Read the model definition and answer for the solid it produces. Units are mm, in the model's axes. A direction names the side the tool comes from. Give positions to 0.01 mm unless a question says otherwise; leave off trailing zeros. Write each loop counter-clockwise with the first axis right and the second up, starting at its lowest first coordinate (ties: lowest second). Pieces come first, ordered by that corner, then holes. Notation, with made-up numbers: (58, 66) - (66, 66) arc R32 ccw to (66, 100) - close; hole circle Ø11 at (-4.75, 76). An arc over 180 degrees is marked (long way). Answer as CSV lines item,"result".
```python
from build123d import *

# Parameters (mm, degrees)
F1_DEPTH      = 15
F2_W          = 70
F2_H          = 12
F3_DEPTH      = 10
F4_R          = 1.375
F4_R_2        = 1
F5_DEPTH      = 25
F5_DEPTH_BACK = 25
F6_R          = 1
F7_DEPTH      = 10


with BuildPart() as f1:
    # F0 (on Top) → F1 (new body)
    with BuildSketch(Plane.XY):
        with BuildLine():
            ThreePointArc((-15.4861029406, 2), (-14.9003165029, 0.5857864376), (-13.4861029406, 0))
            Line((-13.4861029406, 0), (84.5138970594, 0))
            ThreePointArc((84.5138970594, 0), (85.9281106218, 0.5857864376), (86.5138970594, 2))
            Line((86.5138970594, 2), (86.5138970594, 10))
            ThreePointArc((86.5138970594, 10), (85.9281106218, 11.4142135624), (84.5138970594, 12))
            Line((84.5138970594, 12), (-13.4861029406, 12))
            ThreePointArc((-13.4861029406, 12), (-14.9003165029, 11.4142135624), (-15.4861029406, 10))
            Line((-15.4861029406, 10), (-15.4861029406, 2))
        make_face()
    extrude(amount=F1_DEPTH)

    # F2 (on face) → F3 (cut)
    with BuildSketch(Plane.XY.offset(15)):
        with Locations((35.5138970594, 6)):
            Rectangle(F2_W, F2_H)
    extrude(amount=-F3_DEPTH, mode=Mode.SUBTRACT)

    # F4 (on face) → F5 (cut, two sides)
    with BuildSketch(Plane.XY.offset(5)) as f5_sk:
        with Locations((4.5138970594, 8.5)):
            Circle(F4_R)
        with Locations((66.5138970594, 8.5)):
            Circle(F4_R)
        with Locations((-10.4861029406, 4.5)):
            Circle(F4_R_2)
        with Locations((81.5138970594, 4.5)):
            Circle(F4_R_2)
    extrude(amount=-F5_DEPTH, mode=Mode.SUBTRACT)
    extrude(f5_sk.sketch, amount=F5_DEPTH_BACK, mode=Mode.SUBTRACT)

    # F6 (on face) → F7 (cut)
    with BuildSketch(Plane(origin=(0, 0, 0), x_dir=(1, 0, 0), z_dir=(0, 0, -1))):
        with BuildLine():
            Line((76.5138970594, 0), (76.5138970594, -12))
            Line((76.5138970594, -12), (84.5138970594, -12))
            ThreePointArc((84.5138970594, -12), (85.9281106218, -11.4142135624), (86.5138970594, -10))
            Line((86.5138970594, -10), (86.5138970594, -2))
            ThreePointArc((86.5138970594, -2), (85.9281106218, -0.5857864376), (84.5138970594, 0))
            Line((84.5138970594, 0), (76.5138970594, 0))
        make_face()
        with Locations((81.5138970594, -4.5)):
            Circle(F6_R, mode=Mode.SUBTRACT)
        with BuildLine():
            Line((-13.4861029406, -12), (-5.4861029406, -12))
            Line((-5.4861029406, -12), (-5.4861029406, 0))
            Line((-5.4861029406, 0), (-13.4861029406, 0))
            ThreePointArc((-13.4861029406, 0), (-14.9003165029, -0.5857864376), (-15.4861029406, -2))
            Line((-15.4861029406, -2), (-15.4861029406, -10))
            ThreePointArc((-15.4861029406, -10), (-14.9003165029, -11.4142135624), (-13.4861029406, -12))
        make_face()
        with Locations((-10.4861029406, -4.5)):
            Circle(F6_R, mode=Mode.SUBTRACT)
    extrude(amount=-F7_DEPTH, mode=Mode.SUBTRACT)


solid = f1.part
```
(1) For faces 1 (the flat face through (-15.486, 6, 12)), 2 (the flat face through (-5.486, 6, 5)), 3 (the flat face through (70.514, 6, 10)), 4 (the flat face through (86.514, 6, 12)), 5 (the flat face through (76.514, 6, 5)), determine the directions among +Z, -Z, +X, -X, +Y, -Y from which every point of the face is accessible in a straight line to the end or side of a thin tool.
Worked out:
face 1,"+Z, -Z, -X, +Y, -Y"
face 2,"-Z, -X, +Y, -Y"
face 3,"+Z, +Y, -Y"
face 4,"+Z, -Z, +X, +Y, -Y"
face 5,"-Z, +X, +Y, -Y"
(2) A cutting plane is placed at D-D (z = 1.75). Write down the section's boundary in (x, y) (3 decimals).
Worked out:
outline,"(-5.486, 0) - (76.514, 0) - (76.514, 12) - (-5.486, 12) - close; hole circle Ø2.75 at (4.514, 8.5); hole circle Ø2.75 at (66.514, 8.5)"
(3) Each of these flat-tipped pins is pushed along its axis until it touches: P1, Ø3, axis at x = 81.51, y = 4.5, coming from the -Z side; P2, Ø3, axis at y = 7, z = 7.5, coming from the +X side; P3, Ø1, axis at x = 26.5, y = 3.5, coming from the +Z side. Where does it stop, or does it pass through?
Worked out:
P1,"stops at z = 10"
P2,"stops at x = 76.51"
P3,"stops at z = 5"
(4) Find the intervals of material crossed by L1, parallel to X at y = 4.5, z = 11.7; L2, parallel to X at y = 5.25, z = 7.5; L3, parallel to X at y = 2.5, z = 10.25, in increasing order.
Worked out:
L1,"x = -15.49 to -11.49, -9.49 to 0.51, 70.51 to 80.51, 82.51 to 86.51"
L2,"x = -5.49 to 0.51, 70.51 to 76.51"
L3,"x = -15.49 to 0.51, 70.51 to 86.51"
(5) A cutting plane is placed at A-A (z = 12). Write down the section's boundary in (x, y).
Worked out:
outline,"(-15.49, 2) arc R2 ccw to (-13.49, 0) - (0.51, 0) - (0.51, 12) - (-13.49, 12) arc R2 ccw to (-15.49, 10) - close; (70.51, 0) - (84.51, 0) arc R2 ccw to (86.51, 2) - (86.51, 10) arc R2 ccw to (84.51, 12) - (70.51, 12) - close; hole circle Ø2 at (-10.49, 4.5); hole circle Ø2 at (81.51, 4.5)"
(6) A cutting plane is placed at C-C (y = 4.5). Write down the section's boundary in (x, z).
Worked out:
outline,"(-15.49, 10) - (-11.49, 10) - (-11.49, 15) - (-15.49, 15) - close; (-9.49, 10) - (-5.49, 10) - (-5.49, 0) - (76.51, 0) - (76.51, 10) - (80.51, 10) - (80.51, 15) - (70.51, 15) - (70.51, 5) - (0.51, 5) - (0.51, 15) - (-9.49, 15) - close; (82.51, 10) - (86.51, 10) - (86.51, 15) - (82.51, 15) - close"
(7) The mould has two halves that part along Y. Classify faces 6 (the cylindrical face through (-14.885, 11.43, 12.465)), 7 (the flat face through (35, 6, 0)), 8 (the cylindrical face through (4.335, 9.863, 2.535)): +Y half, -Y half, draft (parallel to the pull), parting line (faces both ways), or undercut.
Worked out:
face 6,"+Y half"
face 7,"draft"
face 8,"undercut"
(8) A cutting plane is placed at B-B (y = 8.5). Write down the section's boundary in (x, z), and give its area (4 significant figures).
Worked out:
outline,"(-15.49, 10) - (-5.49, 10) - (-5.49, 0) - (3.14, 0) - (3.14, 5) - (0.51, 5) - (0.51, 15) - (-15.49, 15) - close; (5.89, 0) - (65.14, 0) - (65.14, 5) - (5.89, 5) - close; (67.89, 0) - (76.51, 0) - (76.51, 10) - (86.51, 10) - (86.51, 15) - (70.51, 15) - (70.51, 5) - (67.89, 5) - close"
area,"602.5 mm^2"
